Design review of the part built by this model. Coordinates are the model's own, in mm. Face numbers are marked on the shaded views. A direction names the side the tool comes from. Coordinates: 2 decimals unless noted, no trailing zeros. Loops run counter-clockwise (first coordinate to the right, second up) from the corner with the lowest first, then second, coordinate; pieces in that order, holes last. Notation, with made-up numbers: (-11, -9) - (23, -9) arc R20 ccw to (23, 11) - close; hole circle Ø10 at (5.5, 34.25). An arc over 180 degrees is marked (long way). Return JSON: item names as keys, results as strings. Group by question number.
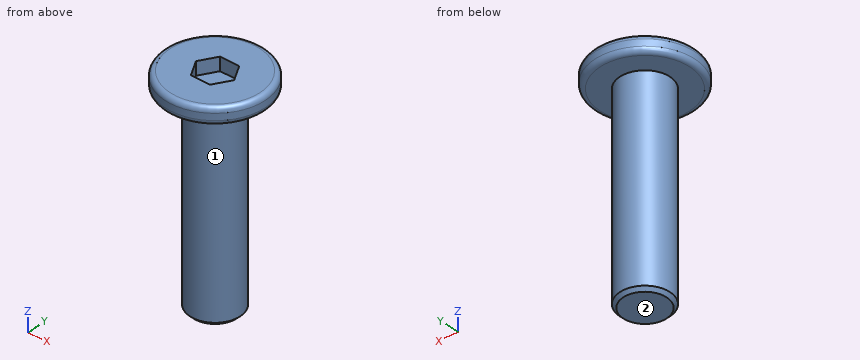
from build123d import *

# Parameters (mm, degrees)
SKETCH_1_R          = 3
EXTRUDE_1_DEPTH     = 0.5
SKETCH_2_R          = 1.5
EXTRUDE_2_DEPTH     = 12
CHAMFER_1_SIZE      = 0.2
CUT_EXTRUDE_1_DEPTH = 0.8
FILLET_2_R          = 0.3


with BuildPart() as part:
    # 草图1 → 凸台-拉伸1 (new body, symmetric)
    with BuildSketch(Plane.XY):
        Circle(SKETCH_1_R)
    extrude(amount=EXTRUDE_1_DEPTH, both=True)

    # 草图2 → 凸台-拉伸2 (add)
    with BuildSketch(Plane(origin=(0, 0, -0.5), x_dir=(-1, 0, 0), z_dir=(0, 0, -1))):
        Circle(SKETCH_2_R)
    extrude(amount=EXTRUDE_2_DEPTH)

    # 倒角1
    chamfer_1_edges = [part.edges().sort_by_distance(p)[0] for p in [
        (1.5, 0, -12.5),
    ]]
    chamfer(chamfer_1_edges, length=CHAMFER_1_SIZE)

    # 草图3 → 切除-拉伸1 (cut)
    with BuildSketch(Plane.XY.offset(0.5)):
        Polygon((1.154700538, 0), (0.577350269, 1), (-0.577350269, 1), (-1.154700538, 0), (-0.577350269, -1), (0.577350269, -1), align=None)
    extrude(amount=-CUT_EXTRUDE_1_DEPTH, mode=Mode.SUBTRACT)

    # 圆角2
    fillet_2_edges = [part.edges().sort_by_distance(p)[0] for p in [
        (-3, 0, -0.5),
        (-3, 0, 0.5),
    ]]
    fillet(fillet_2_edges, radius=FILLET_2_R)


solid = part.part
Item 1: Add section B-B (z = -11). State the section outline as (x, y) points, then the cut area to 3 significant figures.
Item 2: To check wall thickness, follow line 1 (Z direction, x = -1, y = -1.5); line 2 (Y direction, x = -0.75, z = -8). State the ranges of each line that lie inside material, in increasing order. Write a range as from..to.
Item 3: For the marked faces 1 and 2, list the 3-axis set-ups (+Z, -Z, +X, -X, +Y, -Y) from which the entire face can be reached by the end or side of a thin tool; tool diameter is ignored.
Item 4: Add section A-A (x = 0). State the section outline as (y, z) points.
Item 5: For P1, Ø1, axis at x = 0.5, y = -2, coming from the -Z side; P2, Ø3, axis at x = -2, y = -2, coming from the -Z side; P3, Ø1, axis at y = 0, z = -3.5, coming from the +X side; P4, Ø0.9, axis at x = 0.5, z = 0, coming from the -Y side, all flat-tipped, find the tip position at first contact; note any pin that passes through.
Answers below:
{
 "1": {"outline": "circle Ø3 at (0, 0)", "area": "7.07 mm^2"},
 "2": {"line 1": "z = -0.5..0.5", "line 2": "y = -1.3..1.3"},
 "3": {"face 1": "-Z", "face 2": "-Z, +X, -X, +Y, -Y"},
 "4": {"outline": "(-3, -0.2) arc R0.3 ccw to (-2.7, -0.5) - (-1.5, -0.5) - (-1.5, -12.3) - (-1.3, -12.5) - (1.3, -12.5) - (1.5, -12.3) - (1.5, -0.5) - (2.7, -0.5) arc R0.3 ccw to (3, -0.2) - (3, 0.2) arc R0.3 ccw to (2.7, 0.5) - (1, 0.5) - (1, -0.3) - (-1, -0.3) - (-1, 0.5) - (-2.7, 0.5) arc R0.3 ccw to (-3, 0.2) - close"},
 "5": {"P1": "stops at z = -0.5", "P2": "stops at z = -12.47", "P3": "stops at x = 1.5", "P4": "stops at y = -3"}
}
